Autodesk Inventor part; units mm, degrees
ref_plane "YZ Plane" through (0, 0, 0) normal (1, 0, 0) x (0, 1, 0)
ref_plane "XZ Plane" through (0, 0, 0) normal (0, 1, 0) x (-1, 0, 0)
ref_plane "XY Plane" through (0, 0, 0) normal (0, 0, 1) x (1, 0, 0)
sketch "Sketch1" plane through (0, 0, 0) normal (0, 0, 1) x (1, 0, 0)
  line L0 (0, 0) -> (46, 0)
  line L1 (46, 0) -> (46, -25)
  line L2 (46, -25) -> (0, -25)
  line L3 (0, -25) -> (0, 0)
  dimension "d0" = 46
  dimension "d1" = 25
extrude "Extrusion1" add sketch "Sketch1" along normal blind 6
sketch "Sketch2" plane through (0, 0, 6) normal (0, 0, 1) x (1, 0, 0)
  line L0 (46, 0) -> (0, 0) construction
  line L1 (23, 0) -> (23, -25) construction
  line L2 (0, -25) -> (46, -25) construction
  line L3 (0, 0) -> (0, -25) construction
  line L4 (0, -13.8) -> (11.65, -13.8) construction
  point P0 (34.35, -13.8)
  dimension "d5" = 13.8
  dimension "d34" = 11.65
hole "Hole1" at (11.65, -13.8, 6) at (34.35, -13.8, 6) direction (0, 0, -1) diameter 7 end through all
sketch "Sketch3" plane through (0, 0, 6) normal (0, 0, 1) x (1, 0, 0)
  line L0 (46, -25) -> (46, 0)
  line L1 (0, 0) -> (46, 0)
  line L2 (46, 0) -> (46, -6)
  line L3 (46, -6) -> (0, -6)
  line L4 (0, -6) -> (0, 0)
  dimension "d13" = 6
extrude "Extrusion2" add sketch "Sketch3" along normal blind 31.55
sketch "Sketch4" plane through (0, 0, 0) normal (0, 1, 0) x (1, 0, 0)
  line L0 (0, 0) -> (0, -37.55) construction
  line L1 (0, -12.254) -> (5.824, -12.254) construction
  line L2 (0, -6) -> (46, -6) construction
  line L3 (0, 0) -> (46, 0) construction
  line L4 (23, 0) -> (23, -37.55) construction
  line L5 (46, -37.55) -> (0, -37.55) construction
  line L6 (0, -32.254) -> (5.824, -32.254) construction
  point P0 (40.176, -32.254)
  point P1 (40.176, -12.254)
  dimension "d16" = 12.254
  dimension "d17" = 5.824
  dimension "d18" = 20
hole "Hole2" at (5.824, 0, 32.254) at (5.824, 0, 12.254) at (40.176, 0, 32.254) at (40.176, 0, 12.254) direction (0, -1, 0) diameter 4.5 end through all
sketch "Sketch5" plane through (0, -6, 6) normal (0, -1, 0) x (1, 0, 0)
  line L0 (0, 31.55) -> (46, 31.55)
  point P0 (0, -6)
  point P1 (23, 16.55)
  dimension "d26" = 15
hole "Hole3" at (23, -6, 22.55) direction (0, 1, 0) diameter 15 end through all
sketch "Sketch6" plane through (0, 0, 0) normal (0, 1, 0) x (1, 0, 0)
  circle A0 centre (23, -22.55) radius 7.5
  line L0 (0, -37.55) -> (46, -37.55) construction
  line L1 (46, -37.55) -> (0, -37.55) construction
  line L2 (0, -37.55) -> (0, -27.1443) construction
  line L3 (0, 0) -> (0, -37.55) construction
  line L4 (46, -37.55) -> (46, -28.4346) construction
  line L5 (46, -6) -> (46, -37.55) construction
  arc A1 (0, -32.348) -> (3, -37.55) centre (23, -22.55) ccw
  arc A2 (43, -37.55) -> (46, -32.348) centre (23, -22.55) ccw
  line L6 (43, -37.55) -> (46, -37.55)
  line L7 (3, -37.55) -> (0, -37.55)
  line L8 (0, -32.348) -> (0, -37.55)
  line L9 (46, -37.55) -> (46, -32.348)
extrude "Extrusion3" cut sketch "Sketch6" against normal up to next contours A1 L7 L8 | A2 L9 L6
thread "Thread5"
thread "Thread6"
thread "Thread7"
thread "Thread8"
thread "Thread9"
thread "Thread10"
thread "Thread11"
properties part number "X-axis Ball Screw Support"
Here's how the part is built. I have some questions about the finished solid (model axes, mm). A direction names the side the tool comes from. Round coordinates to 2 decimals unless told otherwise and drop trailing zeros. Order: outer loops, then holes, each group sorted by start corner. A loop starts at its lowest first (then second) coordinate and runs counter-clockwise, first axis right, second up. Notation, with made-up numbers: (47.5, -14) -> (51.5, -14) arc R32 ccw to (51.5, 20) -> close; hole circle Ø7 at (-2.5, 71.5). An arc over 180 degrees is marked (long way). Return JSON: item names as keys, results as strings.
Q1. I need wall thicknesses on line 1 along X through (y, z) = (-13.8, 3.05); line 2 along X through (y, z) = (-4, 30.5); line 3 along Z through (x, y) = (23, -4.2). Which ranges of each line are inside material? Lowest first, please. Write a range as from..to.
Filled sheet:
{"line 1": "x = 0..8.15, 15.15..30.85, 37.85..46", "line 2": "x = 0..4.41, 7.23..38.77, 41.59..46", "line 3": "z = 0..15.05, 30.05..37.55"}
Q2. If we section it at C-C on y = -12: List the corners of the cut face in (x, z) for me, plus the area to 3 significant figures.
Filled sheet:
{"outline": "(0, 0) -> (8.65, 0) -> (8.65, 6) -> (0, 6) -> close; (14.65, 0) -> (31.35, 0) -> (31.35, 6) -> (14.65, 6) -> close; (37.35, 0) -> (46, 0) -> (46, 6) -> (37.35, 6) -> close", "area": "204 mm^2"}
Q3. If we section it at A-A on x = 11.65: List the corners of the cut face in (y, z) for me, plus the area to 3 significant figures.
Filled sheet:
{"outline": "(-25, 0) -> (-17.3, 0) -> (-17.3, 6) -> (-25, 6) -> close; (-10.3, 0) -> (0, 0) -> (0, 37.55) -> (-6, 37.55) -> (-6, 6) -> (-10.3, 6) -> close", "area": "297 mm^2"}
Q4. If we mould it in two halves opening along Z, with no side actions, what happens to faces 1 (the flat face through (23, -12, 0)), 2 (the cylindrical face through (7.193, -3.042, 30.468)), 3 (the flat face through (23, 0, 14)), 4 (the flat face through (23, -15, 6))? For each: released by +Z, released by -Z, zero draft, split by the parting line, or undercut.
Filled sheet:
{"face 1": "released by -Z", "face 2": "undercut", "face 3": "zero draft", "face 4": "released by +Z"}
Q5. If we section it at D-D on z = 13: List the corners of the cut face in (x, y) for me, plus the area to 3 significant figures.
Filled sheet:
{"outline": "(0, -6) -> (3.7, -6) -> (3.7, 0) -> (0, 0) -> close; (7.95, -6) -> (38.05, -6) -> (38.05, 0) -> (7.95, 0) -> close; (42.3, -6) -> (46, -6) -> (46, 0) -> (42.3, 0) -> close", "area": "225 mm^2"}
Q6. Which directions (+Z, -Z, +X, -X, +Y, -Y) give clear straight access to the entire face, cutting with the end or side of a thin tool? Please do faces 5 (the flat face through (23, -3, 37.55)), 6 (the flat face through (23.3, -6, 14.5)).
Filled sheet:
{"face 5": "+Z, +X, -X, +Y, -Y", "face 6": "+Z, +X, -X, -Y"}
Q7. For pin 1 Ø5 at (x, z) = (5.824, 12.254) entering from -Y; pin 2 Ø2.5 at (x, z) = (5.824, 32.254) entering from -Y; pin 3 Ø11 at (x, y) = (34.35, -13.8) entering from +Z, each with a flat end and sliding along its axis, tell me the tip position at first contact or that it passes through.
Filled sheet:
{"pin 1": "stops at y = -6", "pin 2": "passes through", "pin 3": "stops at z = 6"}
Q8. If we section it at B-B on z = 19: List the corners of the cut face in (x, y) for me, plus the area to 3 significant figures.
Filled sheet:
{"outline": "(0, -6) -> (16.39, -6) -> (16.39, 0) -> (0, 0) -> close; (29.61, -6) -> (46, -6) -> (46, 0) -> (29.61, 0) -> close", "area": "197 mm^2"}
